Read the model definition and answer for the solid it produces. Units are mm, in the model's axes. A direction names the side the tool comes from. Coordinates: 2 decimals unless noted, no trailing zeros. Loops run counter-clockwise (first coordinate to the right, second up) from the corner with the lowest first, then second, coordinate; pieces in that order, holes last.
Q1. The mould has two halves that part along X. Classify faces 5 (the face through (5, 5, -2)), 6 (the face through (13, 4, -1)), 7 (the face through (0, 1, 1)), 8 (the face through (10.5, 7, -2.7)): pulls with the +X half, pulls with the -X half, needs draft (parallel to the pull), parting line crosses it, or undercut.
Q2. Straight lines are drawn through the part: line 1 (X direction, y = 2.7, z = 0); line 2 (Z direction, x = 0, y = 1.35); line 3 (X direction, y = 0.7, z = 0). For each, find the intervals that lie inside material, in ascending order.
Q3. Section D-D (z = -3.5) is taken. Give the vertices of the cut face in (x, y), then the cut area to 3 significant figures.
Q4. Section B-B (y = 1.75) is taken. Give the vertices of the cut face in (x, z).
Q5. Section A-A (z = 0) is taken. Give the vertices of the cut face in (x, y).
Q6. Flat-ended cylindrical pins translate along their axes: P1, Ø1.2, axis at x = 9, y = 1.5, coming from the +Z side; P2, Ø2, axis at y = 6.5, z = 1, coming from the -X side; P3, Ø1.5, axis at x = 9, z = -3, coming from the +Y side; P4, Ø3.5, axis at x = 0, z = 0, coming from the -Y side. Find the tip coordinate at first contact, or state that the pin passes through.
Q7. Section C-C (x = 7.5) is taken. Give the vertices of the cut face in (y, z).
Q8. Which of the six approach directions +Z, -Z, +X, -X, +Y, -Y give full straight-line access (tool end or side, diameter ignored) to faces 1 (the face through (8, 6, -2)), 2 (the face through (6, 4, 2)), 3 (the face through (11, 2, 3)), 4 (the face through (-1, 2, -1))?
from build123d import *

# Parameters (mm, degrees)
SKETCH1_R           = 1
BOSS_EXTRUDE1_DEPTH = 3
SKETCH2_R           = 3
CUT_EXTRUDE1_DEPTH  = 1
BOSS_EXTRUDE2_DEPTH = 5
CUT_EXTRUDE2_DEPTH  = 13
CUT_EXTRUDE3_DEPTH  = 13


with BuildPart() as part:
    # Sketch1 → Boss-Extrude1 (new body)
    with BuildSketch(Plane(origin=(0, 0, 0), x_dir=(1, 0, 0), z_dir=(0, 1, 0))):
        with BuildLine():
            Line((0, 5), (13, 5))
            Line((13, 5), (13, -3))
            Line((13, -3), (10, -3))
            ThreePointArc((10, -3), (9.414213562, -4.414213562), (8, -5))
            Line((8, -5), (0, -5))
            ThreePointArc((0, -5), (-5, 0), (0, 5))
        make_face()
        Circle(SKETCH1_R, mode=Mode.SUBTRACT)
    extrude(amount=BOSS_EXTRUDE1_DEPTH)

    # Sketch2 → Cut-Extrude1 (cut)
    with BuildSketch(Plane(origin=(0, 3, 0), x_dir=(1, 0, 0), z_dir=(0, 1, 0))):
        Circle(SKETCH2_R)
    extrude(amount=-CUT_EXTRUDE1_DEPTH, mode=Mode.SUBTRACT)

    # Sketch3 → Boss-Extrude2 (add)
    with BuildSketch(Plane(origin=(0, 3, 0), x_dir=(1, 0, 0), z_dir=(0, 1, 0))):
        Polygon((13, -3), (7, -3), (5, -1), (5, 5), (13, 5), align=None)
    extrude(amount=BOSS_EXTRUDE2_DEPTH)

    # Sketch4 → Cut-Extrude2 (cut)
    with BuildSketch(Plane(origin=(13, 0, 0), x_dir=(0, 0, -1), z_dir=(1, 0, 0))):
        Polygon((-3, 4), (1, 8), (-3, 8), align=None)
    extrude(amount=-CUT_EXTRUDE2_DEPTH, mode=Mode.SUBTRACT)

    # Sketch5 → Cut-Extrude3 (cut)
    with BuildSketch(Plane(origin=(0, 0, -5), x_dir=(-1, 0, 0), z_dir=(0, 0, -1))):
        Polygon((-7, 8), (-7, 6), (-10, 6), (-11, 8), align=None)
    extrude(amount=-CUT_EXTRUDE3_DEPTH, mode=Mode.SUBTRACT)


solid = part.part
Numbers:
1. face 5: pulls with the -X half
1. face 6: pulls with the +X half
1. face 7: undercut
1. face 8: undercut
2. line 1: x = -5 to -3, 3 to 13
2. line 2: z = -5 to -1, 1 to 5
2. line 3: x = -5 to -1, 1 to 13
3. outline: (-3.57, 0) - (13, 0) - (13, 8) - (11, 8) - (10, 6) - (7, 6) - (7, 8) - (5, 8) - (5, 3) - (-3.57, 3) - close
3. area: 82.7 mm2
4. outline: (0, -5) - (13, -5) - (13, 3) - (10, 3) arc R2 ccw to (8, 5) - (0, 5) arc R5 ccw to start; hole circle Ø2 at (0, 0)
5. outline: (-5, 0) - (-1, 0) - (-1, 2) - (-3, 2) - (-3, 3) - (-5, 3) - close; (1, 0) - (13, 0) - (13, 7) - (10.5, 7) - (10, 6) - (7, 6) - (7, 7) - (5, 7) - (5, 3) - (3, 3) - (3, 2) - (1, 2) - close
6. P1: stops at z = 4.96
6. P2: stops at x = 5
6. P3: stops at y = 6
6. P4: stops at y = 0
7. outline: (0, -5) - (6, -5) - (6, 1) - (4, 3) - (3, 3) - (3, 5) - (0, 5) - close
8. face 1: +Z, -Z, +Y
8. face 2: +Z, -X, +Y
8. face 3: +Z, +X, +Y
8. face 4: +Y
